Source: CAD feature listing. Evaluate the final solid. Frame: model axes, mm. A direction names the side the tool comes from. Round coordinates to 2 decimals unless told otherwise and drop trailing zeros. Write each loop counter-clockwise with the first axis right and the second up, starting at its lowest first coordinate (ties: lowest second). Pieces come first, ordered by that corner, then holes. Notation, with made-up numbers: (34, -29) -> (75, -29) arc R31 cw to (75, 0) -> close; hole circle Ø8 at (-25, -12). An arc over 180 degrees is marked (long way). Put each result on its own line as item: value.
```python
from build123d import *

# Parameters (mm, degrees)
F1_DEPTH       = 3.81
F2_DEPTH       = 3.302
F4_D           = 1.524
F4_CSINK_D     = 7.112
F4_CSINK_ANGLE = 90
F6_DEPTH       = 1.016
F7_W           = 1.778
F7_H           = 3.556
F8_DEPTH       = 0.508
F9_W           = 3.302
F9_H           = 3.556
F10_DEPTH      = 0.508
F11_W          = 3.302
F11_H          = 3.556
F12_DEPTH      = 0.508
F13_R          = 0.396875
F13_R_2        = 0.3737664599
F14_DEPTH      = 1.27


with BuildPart() as f1:
    # F0 (on Front) → F1 (new body)
    with BuildSketch(Plane.XZ):
        Polygon((21.3439739875, 15.0127133582), (11.1839739875, 15.0127133582), (11.1839739875, -7.8472866418), (11.6919739875, -7.8472866418), (20.8359739875, -7.8472866418), (21.3439739875, -7.8472866418), align=None)
    extrude(amount=F1_DEPTH)

    # F0 (on Front) → F2 (join)
    with BuildSketch(Plane.XZ):
        Polygon((20.8359739875, -7.8472866418), (11.6919739875, -7.8472866418), (11.6919739875, -11.1442380585), (12.9619739875, -12.4142380585), (19.5659739875, -12.4142380585), (20.8359739875, -11.1442380585), align=None)
    extrude(amount=F2_DEPTH)

    # F4 (through all)
    with Locations(Plane.XZ.offset(3.81)):
        with Locations((16.2639739875, 9.9327133582)):
            CounterSinkHole(F4_D / 2, F4_CSINK_D / 2, counter_sink_angle=F4_CSINK_ANGLE)

    # F5 (on face) → F6 (cut)
    with BuildSketch(Plane.XZ.offset(3.81)):
        Polygon((16.6935976049, 4.5998531383), (16.1855976049, 4.5998531383), (15.6775976049, 4.5998531383), (15.6775976049, -1.7501468617), (16.6935976049, -1.7501468617), align=None)
    extrude(amount=-F6_DEPTH, mode=Mode.SUBTRACT)

    # F7 (on face) → F8 (cut)
    with BuildSketch(Plane.XZ.offset(3.81)):
        with Locations((12.0729739875, -4.2912866418)):
            Rectangle(F7_W, F7_H)
        with Locations((20.4549739875, -4.2912866418)):
            Rectangle(F7_W, F7_H)
    extrude(amount=-F8_DEPTH, mode=Mode.SUBTRACT)

    # F9 (on face) → F10 (cut)
    with BuildSketch(Plane.YZ.offset(21.3439739875)):
        with Locations((-1.651, -4.2912866418)):
            Rectangle(F9_W, F9_H)
    extrude(amount=-F10_DEPTH, mode=Mode.SUBTRACT)

    # F11 (on face) → F12 (cut)
    with BuildSketch(Plane(origin=(11.1839739875, 0, 0), x_dir=(0, -1, 0), z_dir=(-1, 0, 0))):
        with Locations((1.651, -4.2912866418)):
            Rectangle(F11_W, F11_H)
    extrude(amount=-F12_DEPTH, mode=Mode.SUBTRACT)

    # F13 (on face) → F14 (cut)
    with BuildSketch(Plane.XZ.offset(3.302)):
        with Locations((13.0889739875, -9.3712866418)):
            Circle(F13_R)
        with Locations((14.6764739875, -9.3712866418)):
            Circle(F13_R)
        with Locations((13.8395041891, -10.1650366418)):
            Circle(F13_R)
        with Locations((15.4270041891, -10.1650366418)):
            Circle(F13_R)
        with Locations((16.2639739875, -9.3712866418)):
            Circle(F13_R_2)
        with Locations((17.1009437859, -10.1650366418)):
            Circle(F13_R)
        with Locations((17.8514739875, -9.3712866418)):
            Circle(F13_R)
        with Locations((18.6884437859, -10.1650366418)):
            Circle(F13_R)
        with Locations((19.4389739875, -9.3712866418)):
            Circle(F13_R)
    extrude(amount=-F14_DEPTH, mode=Mode.SUBTRACT)


solid = f1.part
```
Q1. Reachability of faces 5 (the flat face through (15.9, -3.6, -7.847)), 6 (the flat face through (16, -3, 4.6)), 7 (the flat face through (11.5, -2.3, -2.513)), 8 (the flat face through (11.692, -2, -4)), 9 (the flat face through (16, -3.302, -10)) from +Z, -Z, +X, -X, +Y, -Y: full face, straight path, thin tool, end or side. Return the list, or none.
Ans:
face 5: -Z, -Y
face 6: -Y
face 7: -X, -Y
face 8: -X, +Y, -Y
face 9: -Z, +X, -X, -Y
Q2. Pin query (flat end, axial travel): pin 1 (1.4 mm diameter, centred on x = 11.5, y = -1, fed in from -Z); pin 2 (0.9 mm diameter, centred on x = 20.5, y = -1.5, fed in from -Z); pin 3 (0.6 mm diameter, centred on y = -3.5, z = -3.5, fed in from +X). Return the tip coordinate at first contact, or that it passes through.
Ans:
pin 1: stops at z = -11.65
pin 2: stops at z = -11.93
pin 3: stops at x = 20.84
Q3. Cut plane B-B on z = -5. Output: boundary loops of the cut face in (x, y).
Ans:
outline: (11.69, -3.3) -> (12.96, -3.3) -> (12.96, -3.81) -> (19.57, -3.81) -> (19.57, -3.3) -> (20.84, -3.3) -> (20.84, 0) -> (11.69, 0) -> close
Q4. Cut plane D-D on x = 20.5. Output: boundary loops of the cut face in (y, z), and give its area (3 significant figures).
Ans:
outline: (-3.81, -7.85) -> (-3.3, -7.85) -> (-3.3, -11.48) -> (0, -11.48) -> (0, 15.01) -> (-3.81, 15.01) -> (-3.81, -2.51) -> (-3.3, -2.51) -> (-3.3, -6.07) -> (-3.81, -6.07) -> close
area: 97.3 mm^2
Q5. Material intervals for line 1 (Z direction, x = 19.5, y = -2.4); line 2 (Z direction, x = 20, y = -3.55); line 3 (X direction, y = -2.95, z = -10), sorted ascending. Write a range as [from, to].
Ans:
line 1: z = [-12.41, -9.76], [-8.98, 15.01]
line 2: z = [-7.85, -6.07], [-2.51, 15.01]
line 3: x = [11.69, 13.48], [14.2, 15.07], [15.79, 16.74], [17.46, 18.33], [19.05, 20.84]
Q6. Draft query along X for faces 1 (the flat face through (21, -2, -6.069)), 2 (the flat face through (16, -3, -1.75)), 3 (the flat face through (21.344, -2, -7)), 4 (the flat face through (12.32, -1.63, -11.77)). Return one class per face: +X half, -X half, draft (parallel to the pull), parting line (faces both ways), or undercut.
Ans:
face 1: draft
face 2: undercut
face 3: +X half
face 4: -X half
Q7. Cut plane A-A on y = -2.55. Give the number of separate pieces and of enclosed holes in the cut face, and give its area (3 significant figures).
Ans:
separate pieces: 1
enclosed holes: 10
area: 248 mm^2
Q8. Cut plane C-C on y = -0.3. Output: boundary loops of the cut face in (x, z), and give its area (3 significant figures).
Ans:
outline: (11.18, -7.85) -> (11.69, -7.85) -> (11.69, -11.14) -> (12.96, -12.41) -> (19.57, -12.41) -> (20.84, -11.14) -> (20.84, -7.85) -> (21.34, -7.85) -> (21.34, -6.07) -> (20.84, -6.07) -> (20.84, -2.51) -> (21.34, -2.51) -> (21.34, 15.01) -> (11.18, 15.01) -> (11.18, -2.51) -> (11.69, -2.51) -> (11.69, -6.07) -> (11.18, -6.07) -> close; hole circle Ø1.52 at (16.26, 9.93)
area: 267 mm^2
